Autodesk Inventor part; units mm, degrees
ref_plane "YZ Plane" through (0, 0, 0) normal (1, 0, 0) x (0, 1, 0)
ref_plane "XZ Plane" through (0, 0, 0) normal (0, 1, 0) x (-1, 0, 0)
ref_plane "XY Plane" through (0, 0, 0) normal (0, 0, 1) x (1, 0, 0)
sketch "Sketch1" plane through (0, 0, 0) normal (0, 1, 0) x (-1, 0, 0)
  line L0 (-9.5451, 18.566) -> (9.5451, 18.566)
  line L1 (9.5451, 18.566) -> (9.5451, -18.566)
  line L2 (9.5451, -18.566) -> (-9.5451, -18.566)
  line L3 (-9.5451, -18.566) -> (-9.5451, 18.566)
  line L4 (-9.5451, 18.566) -> (9.5451, -18.566) construction
  line L5 (9.5451, 18.566) -> (-9.5451, -18.566) construction
  line L6 (-5.4388, 18.566) -> (5.4388, 18.566)
  line L7 (5.4388, 18.566) -> (5.4388, -18.566)
  line L8 (5.4388, -18.566) -> (-5.4388, -18.566)
  line L9 (-5.4388, -18.566) -> (-5.4388, 18.566)
  line L10 (-5.4388, 18.566) -> (5.4388, -18.566) construction
  line L11 (5.4388, 18.566) -> (-5.4388, -18.566) construction
  point P0 (0, 0)
extrude "Extrusion1" add sketch "Sketch1" along normal blind 10 contours L0 L9 L2 L3 | L0 L1 L2 L7
extrude "Extrusion2" add sketch "Sketch1" against normal blind 4.5
sketch "Sketch2" plane through (9.5451, 10, 18.566) normal (1, 0, 0) x (0, 0, -1)
  line L0 (3.8006, -2.9012) -> (31.8899, -2.9012)
  point P0 (18.566, -10)
hole "Hole1" at (9.5451, 7.0988, 14.7655) at (9.5451, 7.0988, -13.3239) direction (-1, 0, 0) diameter 3.2 end through all
Input: part model. Units: mm. Frame: model coordinates. A direction names the side the tool comes from. Coordinates: 2 decimals unless noted, no trailing zeros. Loops run counter-clockwise (first coordinate to the right, second up) from the corner with the lowest first, then second, coordinate; pieces in that order, holes last. Notation, with made-up numbers: M 56,70 L 107,70 A35 ccw 107,109 Z; hole C -28.5,-36.75 d3. An arc over 180 degrees is marked long. Use a Markdown table: item, result. Add a question column.
1) Line query: L1, parallel to X at y = 2, z = -14; L2, parallel to Z at x = -5.5, y = 8.5; L3, parallel to Y at x = 8.75, z = 14. Output: solid intervals per line, ascending. Write a range as from..to.
2) Section D-D, the plane x = -6.5. Return the cut outline in (y, z), plus the area to 3 significant figures.
3) Section C-C, the plane y = 8. Return the cut outline in (x, z).
4) Draft query along Y for faces 3 (the flat face through (0, -4.5, 0)), 4 (the cylindrical face through (-7.521, 7.712, -14.802)), 5 (the flat face through (8, 10, 0)). Return one class per face: +Y half, -Y half, draft (parallel to the pull), parting line (faces both ways), or undercut.
5) Pin query (flat end, axial travel): P1, Ø3, axis at y = 7.1, z = 14.77, coming from the +X side; P2, Ø3.5, axis at x = 2, z = -2, coming from the +Y side. Return the tip coordinate at first contact, or that it passes through.
6) Set-up query: faces 1 (the cylindrical face through (7.463, 7.712, -14.802)), 2 (the flat face through (-5.439, 5, 0)). Return all of +Z, -Z, +X, -X, +Y, -Y with unobstructed straight access to the full face (end or side cutting, diameter ignored); none if empty.
7) Section B-B, the plane z = -3. Return the cut outline in (x, y), plus the area to 3 significant figures.
8) Section A-A, the plane y = 3.25. Return the cut outline in (x, z).
Answer below:
| question | item | result |
|---|---|---|
| 1 | L1 | -9.55..-5.44, 5.44..9.55 |
| 1 | L2 | -18.57..-14.1, -12.55..13.99, 15.54..18.57 |
| 1 | L3 | -4.5..5.69, 8.5..10 |
| 2 | outline | M -4.5,-18.57 L 10,-18.57 L 10,18.57 L -4.5,18.57 Z; hole C 7.1,-13.32 d3.2; hole C 7.1,14.77 d3.2 |
| 2 | area | 522 mm2 |
| 3 | outline | M -9.55,-18.57 L -5.44,-18.57 L -5.44,-14.65 L -9.55,-14.65 Z; M -9.55,-12 L -5.44,-12 L -5.44,13.44 L -9.55,13.44 Z; M -9.55,16.09 L -5.44,16.09 L -5.44,18.57 L -9.55,18.57 Z; M 5.44,-18.57 L 9.55,-18.57 L 9.55,-14.65 L 5.44,-14.65 Z; M 5.44,-12 L 9.55,-12 L 9.55,13.44 L 5.44,13.44 Z; M 5.44,16.09 L 9.55,16.09 L 9.55,18.57 L 5.44,18.57 Z |
| 4 | face 3 | -Y half |
| 4 | face 4 | undercut |
| 4 | face 5 | +Y half |
| 5 | P1 | through |
| 5 | P2 | y = 0 |
| 6 | face 1 | +X, -X |
| 6 | face 2 | +Z, -Z, +Y |
| 7 | outline | M -9.55,-4.5 L 9.55,-4.5 L 9.55,10 L 5.44,10 L 5.44,0 L -5.44,0 L -5.44,10 L -9.55,10 Z |
| 7 | area | 168 mm2 |
| 8 | outline | M -9.55,-18.57 L -5.44,-18.57 L -5.44,18.57 L -9.55,18.57 Z; M 5.44,-18.57 L 9.55,-18.57 L 9.55,18.57 L 5.44,18.57 Z |
